The model under review builds one solid part; all positions refer to its coordinate system, in mm. A direction names the side the tool comes from. Coordinates: 2 decimals unless noted, no trailing zeros. Order: outer loops, then holes, each group sorted by start corner. A loop starts at its lowest first (then second) coordinate and runs counter-clockwise, first axis right, second up. Notation, with made-up numbers: (20.5, -27) -> (46.5, -27) arc R12 cw to (46.5, -23) -> close; hole circle Ø1 at (-26, -39). An arc over 180 degrees is marked (long way). Answer as CSV lines item,"result". Start each with the question number.
from build123d import *

# Parameters (mm, degrees)
CROQUIS1_W              = 30
CROQUIS1_H              = 33
SALIENTE_EXTRUIR1_DEPTH = 95
CROQUIS2_R              = 2
CORTAR_EXTRUIR1_DEPTH   = 5


with BuildPart() as part:
    # Croquis1 → Saliente-Extruir1 (new body)
    with BuildSketch(Plane.XY):
        Rectangle(CROQUIS1_W, CROQUIS1_H)
    extrude(amount=-SALIENTE_EXTRUIR1_DEPTH)

    # Croquis2 → Cortar-Extruir1 (cut)
    with BuildSketch(Plane(origin=(0, 16.5, 0), x_dir=(1, 0, 0), z_dir=(0, 1, 0))):
        with Locations(Location((0, 16, 0), (0, 0, 180))):
            Circle(CROQUIS2_R)
        with Locations((0, 79)):
            Circle(CROQUIS2_R)
    extrude(amount=-CORTAR_EXTRUIR1_DEPTH, mode=Mode.SUBTRACT)


solid = part.part
1) Consider section A-A (z = -16). Give the boundary of the cut face in (x, y).
2) Insertion check: pin 1 Ø2 at (x, z) = (-0.5, -79.5) entering from +Y. The pin has a flat end and moves straight along its axis. Give the tip position at first contact, or say it passes through.
3) Wall thickness on L1, parallel to Z at x = 0, y = 13.5; L2, parallel to X at y = 14.7, z = -79; L3, parallel to Z at x = 1.5, y = 15.5: over which ranges is each line inside the solid? List them lowest first. Write a range as [from, to].
4) Mouldability with a two-part tool opening along X and no side actions: class faces 1 (the face through (0, -16.5, -47)), 2 (the face through (15, 0, -47)), 3 (the face through (0, 14, -14)) as released by +X, released by -X, zero draft, split by the parting line, or undercut.
5) Tool access review of faces 4 (the face through (0, 16.5, -47)), 5 (the face through (0, 11.5, -16)): name each direction out of +Z, -Z, +X, -X, +Y, -Y from which nothing blocks a thin tool from reaching the whole face with its end or side.
Result:
1,outline,"(-15, -16.5) -> (15, -16.5) -> (15, 16.5) -> (2, 16.5) -> (2, 11.5) -> (-2, 11.5) -> (-2, 16.5) -> (-15, 16.5) -> close"
2,pin 1,"y = 11.5"
3,L1,"[-95, -81], [-77, -18], [-14, 0]"
3,L2,"[-15, -2], [2, 15]"
3,L3,"[-95, -80.32], [-77.68, -17.32], [-14.68, 0]"
4,face 1,"zero draft"
4,face 2,"released by +X"
4,face 3,"undercut"
5,face 4,"+Z, -Z, +X, -X, +Y"
5,face 5,"+Y"
